Geometry: final body of the model. Coordinates: model frame, mm. Give positions to 0.01 mm unless a question says otherwise; leave off trailing zeros. Loops run counter-clockwise (first coordinate to the right, second up) from the corner with the lowest first, then second, coordinate; pieces in that order, holes last. Notation, with made-up numbers: (-8.5, -33.5) -> (49.5, -33.5) arc R19 ccw to (49.5, -18.5) -> close; hole circle Ø1 at (-34, 45.25). An arc over 180 degrees is marked (long way). One line per question, with ' | ' between items. Start each with the question number.
Item 1: Section A-A on x = 0. Return loops of the section in (y, z), then the cut area to 3 significant figures.
Item 2: Material intervals for line 1 along Z through (x, y) = (3.5, 1.5); line 2 along Y through (x, z) = (0, 7.2); line 3 along Y through (x, z) = (-0.5, 5.75), sorted ascending. Write a range as [from, to].
Item 3: Section C-C on z = 3.25. Return loops of the section in (x, y), then the cut area to 3 significant figures.
Item 4: Pin query (flat end, axial travel): P1, Ø2, axis at x = 0, y = 2.5, coming from the -Z side; P2, Ø4, axis at x = 2.5, z = -1.5, coming from the -Y side; P3, Ø2, axis at x = 1.5, z = 2.5, coming from the +Y side. Return the tip coordinate at first contact, or that it passes through.
Item 5: Mould query, pull axis X, two halves, no side actions, for faces 1 (the cylindrical face through (-6, 0, 4)), 2 (the flat face through (-0.1, 1.4, 8.5)), 3 (the flat face through (0, 0, 5.5)). Classes: released by +X, released by -X, zero draft, split by the parting line, or undercut.
Item 6: Section B-B on z = -0.25. Return loops of the section in (x, y).
Autodesk Fusion 360 part; units mm, degrees
sketch "Sketch1" plane through (0, 0, 0) normal (0, 0, 1) x (1, 0, 0)
  circle A0 centre (0, 0) radius 6
  circle A1 centre (0, 0) radius 1.25
  line L0 (-6, 0.0236) -> (6, 0.0236) construction
  line L1 (-6, 0.0236) -> (-3.5, 0.0236) construction
  line L2 (6, 0.0236) -> (3.5, 0.0236) construction
  circle A2 centre (3.5, 0.0236) radius 0.3
  circle A3 centre (-3.5, 0.0236) radius 0.3
  dimension "d1" = 12
  dimension "d2" = 2.5
  dimension "d3" = 2.5
  dimension "d5" = 2.5
  dimension "d6" = 0.6
  dimension "d7" = 0.6
extrude "Extrude1" add sketch "Sketch1" along normal blind 8.5 contours A0 | A1 | A2 | A3
sketch "Sketch2" plane through (0, 0, 8.5) normal (0, 0, 1) x (-1, 0, 0)
  circle A0 centre (0, 0) radius 6
  circle A1 centre (0, 0) radius 1.25
  circle A2 centre (4.0974, 0) radius 1.25
  line L0 (3.9724, 0.75) -> (4.2224, 0.75)
  line L1 (4.2224, 0.75) -> (4.2224, -0.75)
  line L2 (4.2224, -0.75) -> (3.9724, -0.75)
  line L3 (3.9724, -0.75) -> (3.9724, 0.75)
  line L4 (3.9724, 0.75) -> (4.2224, -0.75) construction
  line L5 (4.2224, 0.75) -> (3.9724, -0.75) construction
  line L6 (4.8474, -0.125) -> (3.3474, -0.125)
  line L7 (4.8474, 0.125) -> (4.8474, -0.125)
  line L8 (3.3474, 0.125) -> (4.8474, 0.125)
  line L9 (3.3474, -0.125) -> (3.3474, 0.125)
  point P0 (4.0974, 0)
  dimension "d14" = 2.5
  dimension "d15" = 1.5
  dimension "d16" = 0.25
  dimension "d18" = 90
extrude "Extrude4" cut sketch "Sketch2" against normal blind 0.1 contours A2
extrude "Extrude2" cut sketch "Sketch2" against normal blind 3 contours A1
extrude "Extrude3" add sketch "Sketch1" against normal blind 5.5 contours A2 | A3
fillet "Fillet1" radius 0.25 1 edges at (-5.594, -2.1697, 8.5)
Result sheet:
1) outline: (-6, 0) -> (6, 0) -> (6, 8.25) arc R0.25 ccw to (5.75, 8.5) -> (1.25, 8.5) -> (1.25, 5.5) -> (-1.25, 5.5) -> (-1.25, 8.5) -> (-5.75, 8.5) arc R0.25 ccw to (-6, 8.25) -> close | area: 94.5 mm²
2) line 1: z = [0, 8.5] | line 2: y = [-6, -1.25], [1.25, 6] | line 3: y = [-5.98, -1.15], [1.15, 5.98]
3) outline: circle Ø12 at (0, 0) | area: 113 mm²
4) P1: stops at z = 0 | P2: stops at y = -5.88 | P3: stops at y = 5.98
5) face 1: split by the parting line | face 2: zero draft | face 3: undercut
6) outline: circle Ø0.6 at (-3.5, 0.02); circle Ø0.6 at (3.5, 0.02)
